from build123d import *

# Parameters (mm, degrees)
SKETCH2_R           = 30
BOSS_EXTRUDE1_DEPTH = 5
SKETCH3_R           = 15
BOSS_EXTRUDE2_DEPTH = 19.05
CUT_EXTRUDE1_DEPTH  = 24.05
SKETCH5_R           = 2
BOSS_EXTRUDE3_DEPTH = 2


with BuildPart() as part:
    # Sketch2 → Boss-Extrude1 (new body)
    with BuildSketch(Plane(origin=(0, 0, 0), x_dir=(0, 0, -1), z_dir=(1, 0, 0))):
        Circle(SKETCH2_R)
    extrude(amount=BOSS_EXTRUDE1_DEPTH)

    # Sketch3 → Boss-Extrude2 (add)
    with BuildSketch(Plane(origin=(5, 0, 0), x_dir=(0, 0, -1), z_dir=(1, 0, 0))):
        with Locations(Location((0, 0, 0), (0, 0, 180))):
            Circle(SKETCH3_R)
    extrude(amount=BOSS_EXTRUDE2_DEPTH)

    # Sketch4 → Cut-Extrude1 (cut)
    with BuildSketch(Plane(origin=(24.05, 0, 0), x_dir=(0, 0, -1), z_dir=(1, 0, 0))):
        Polygon((0, 5.64071213), (-4.885, 2.820356065), (-4.885, -2.820356065), (0, -5.64071213), (4.885, -2.820356065), (4.885, 2.820356065), align=None)
    extrude(amount=-CUT_EXTRUDE1_DEPTH, mode=Mode.SUBTRACT)

    # Sketch5 → Boss-Extrude3 (add)
    with BuildSketch(Plane(origin=(24.05, 0, 0), x_dir=(0, 0, -1), z_dir=(1, 0, 0))):
        with Locations((8.937690528, 5.160178032)):
            Circle(SKETCH5_R)
        with Locations((-8.937690528, 5.160178032)):
            Circle(SKETCH5_R)
        with Locations((0, -10.320356065)):
            Circle(SKETCH5_R)
    extrude(amount=BOSS_EXTRUDE3_DEPTH)


solid = part.part
The model under review builds one solid part; all positions refer to its coordinate system, in mm. A direction names the side the tool comes from. Give positions to 0.01 mm unless a question says otherwise; leave off trailing zeros. Loops run counter-clockwise (first coordinate to the right, second up) from the corner with the lowest first, then second, coordinate; pieces in that order, holes last. Notation, with made-up numbers: (61.5, 45) -> (68.5, 45) arc R13 cw to (68.5, 62) -> close; hole circle Ø8 at (-11.75, 16.5). An arc over 180 degrees is marked (long way). Answer as a JSON object with one key per item and string values. Group by question number.
Q1. Wall thickness on line 1 along X through (y, z) = (13, -0.5); line 2 along Z through (x, y) = (4.5, 3.5); line 3 along X through (y, z) = (-21, 4): over which ranges is each line inside the solid? List them lowest first.
Q2. Tool access review of faces 4 (the flat face through (12.19, 4.21, -2.48)), 5 (the flat face through (0, 0, -6)), 6 (the cylindrical face through (25.036, 5.761, -10.845)): name each direction out of +Z, -Z, +X, -X, +Y, -Y from which nothing blocks a thin tool from reaching the whole face with its end or side.
Q3. Insertion check: pin 1 (8 mm diameter, centred on y = 22, z = 12, fed in from +X); pin 2 (10 mm diameter, centred on x = 5, y = -15.5, fed in from -Z); pin 3 (2 mm diameter, centred on x = 13, y = -0.5, fed in from -Z). Each pin has a flat end and moves straight along its axis. Give the tip position at first contact, or say it passes through.
Q4. Take a section at C-C (z = -6). Write out the cut boundary in (x, y).
Q5. Take a section at D-D (y = 23.5). Write out the cut boundary in (x, z).
Q6. Take a section at B-B (x = 17). Write out the cut boundary in (y, z) (3 decimals), plus the area to 3 significant figures.
Q7. Draft analysis for pull direction Z (two halves, no side actions). For faces 1 (the cylindrical face through (25.036, -8.337, 0.26)), 2 (the flat face through (12.19, 4.25, 2.41)), 3 (the flat face through (26.05, 5, -9)), state which applies: pulls with the +Z half, pulls with the -Z half, needs draft (parallel to the pull), parting line crosses it, or undercut.
Q8. Take a section at A-A (y = 0). Write out the cut boundary in (x, z) (3 decimals).
Answer below:
{
 "1": {"line 1": "x = 0 to 24.05", "line 2": "z = -29.8 to -3.71, 3.71 to 29.8", "line 3": "x = 0 to 5"},
 "2": {"face 4": "+X, -X", "face 5": "+Z, -Z, -X, +Y, -Y", "face 6": "+X"},
 "3": {"pin 1": "stops at x = 5", "pin 2": "stops at z = -28.1", "pin 3": "stops at z = -15"},
 "4": {"outline": "(0, -29.39) -> (5, -29.39) -> (5, -13.75) -> (24.05, -13.75) -> (24.05, 13.75) -> (5, 13.75) -> (5, 29.39) -> (0, 29.39) -> close"},
 "5": {"outline": "(0, -18.65) -> (5, -18.65) -> (5, 18.65) -> (0, 18.65) -> close"},
 "6": {"outline": "circle Ø30 at (0, 0); hole (-5.641, 0) -> (-2.82, -4.885) -> (2.82, -4.885) -> (5.641, 0) -> (2.82, 4.885) -> (-2.82, 4.885) -> close", "area": "624 mm2"},
 "7": {"face 1": "parting line crosses it", "face 2": "undercut", "face 3": "needs draft"},
 "8": {"outline": "(0, -30) -> (5, -30) -> (5, -15) -> (24.05, -15) -> (24.05, -4.885) -> (0, -4.885) -> close; (0, 4.885) -> (24.05, 4.885) -> (24.05, 15) -> (5, 15) -> (5, 30) -> (0, 30) -> close"}
}
